Autodesk Inventor part; units mm, degrees
ref_plane "Work Plane1" through (17.5, 0, 4) normal (1, 0, 0) x (0, 0, -1)
ref_plane "YZ Plane" through (0, 0, 0) normal (1, 0, 0) x (0, 1, 0)
ref_plane "XZ Plane" through (0, 0, 0) normal (0, 1, 0) x (-1, 0, 0)
sketch "Sketch1" plane through (0, 0, 0) normal (0, 0, 1) x (1, 0, 0)
  line L0 (0, 0) -> (35, 0)
  line L1 (35, 0) -> (35, 55)
  line L2 (35, 55) -> (0, 55)
  line L3 (0, 55) -> (0, 0)
  dimension "d0" = 35
  dimension "d1" = 55
extrude "Extrusion1" add sketch "Sketch1" along normal mid plane 8
sketch "Sketch2" plane through (35, 0, 4) normal (1, 0, 0) x (0, 0, -1)
  line L0 (8, 55) -> (0, 55)
  point P0 (4, 0)
  point P1 (4, 7.5)
  point P2 (4, 47.5)
  point P3 (4, 55)
  dimension "d4" = 7.5
  dimension "d5" = 7.5
  dimension "d6" = 40
hole "Hole1" at (35, 7.5, 0) at (35, 47.5, 0) direction (-1, 0, 0) diameter 2.459 depth 8.8 tip angle 118
ref_plane "Work Plane1" through (17.5, 0, 4) normal (1, 0, 0) x (0, 0, -1)
mirror "Mirror1" about plane through (17.5, 0, 4) normal (1, 0, 0) of "Hole1"
properties part number "Pancake_Floor Piece" material "Aluminum 6061"
For this review, take the finished solid that the model builds, in its own axes (mm). A direction names the side the tool comes from. Round coordinates to 2 decimals unless told otherwise and drop trailing zeros. Loops run counter-clockwise (first coordinate to the right, second up) from the corner with the lowest first, then second, coordinate; pieces in that order, holes last. Notation, with made-up numbers: (-24, -11) - (32, -11) arc R26 ccw to (32, 11) - close; hole circle Ø3 at (64, 48.5). An arc over 180 degrees is marked (long way). Answer as CSV lines item,"result".
(1) Wall thickness on line 1 (Y direction, x = 7.25, z = 0); line 2 (Y direction, x = 28, z = 0.5); line 3 (Z direction, x = 3.75, y = 7.5): over which ranges is each line inside the solid? List them lowest first.
Checked values:
line 1,"y = 0 to 6.27, 8.73 to 46.27, 48.73 to 55"
line 2,"y = 0 to 6.38, 8.62 to 46.38, 48.62 to 55"
line 3,"z = -4 to -1.23, 1.23 to 4"
(2) Consider section A-A on x = 6. Give the boundary of the cut face in (y, z).
Checked values:
outline,"(0, -4) - (55, -4) - (55, 4) - (0, 4) - close; hole circle Ø2.46 at (7.5, 0); hole circle Ø2.46 at (47.5, 0)"
(3) Tool access review of faces 5 (the face through (35, 27, 0)), 6 (the face through (30.54, 8.7, 0.27)), 7 (the face through (4.46, 48.72, 0.16)): name each direction out of +Z, -Z, +X, -X, +Y, -Y from which nothing blocks a thin tool from reaching the whole face with its end or side.
Checked values:
face 5,"+Z, -Z, +X, +Y, -Y"
face 6,"+X"
face 7,"-X"
(4) Mouldability with a two-part tool opening along Z and no side actions: class faces 1 (the face through (9.41, 7.71, 0.05)), 2 (the face through (17, 28, -4)), 3 (the face through (0, 28, 0)), 4 (the face through (17, 28, 4)) as +Z half, -Z half, draft (parallel to the pull), parting line (faces both ways), or undercut.
Checked values:
face 1,"undercut"
face 2,"-Z half"
face 3,"draft"
face 4,"+Z half"
(5) Insertion check: P1, Ø2, axis at y = 47.5, z = 0, coming from the -X side. The pin has a flat end and moves straight along its axis. Give the tip position at first contact, or say it passes through.
Checked values:
P1,"stops at x = 8.94"
